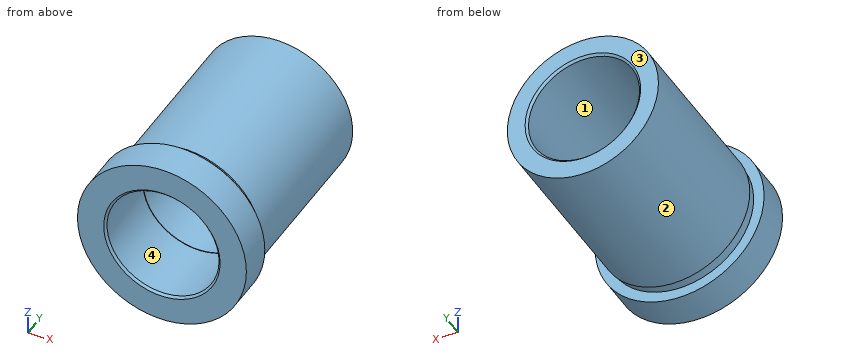
from build123d import *

# Parameters (mm, degrees)
CUT_EXTRUDE1_DEPTH      = 57.762663785
CUT_EXTRUDE1_DEPTH_BACK = 57.762663785
SKETCH2_R               = 12.5
SKETCH4_R               = 12.6
CUT_EXTRUDE2_DEPTH      = 16
CHAMFER4_SIZE           = 0.5
CHAMFER5_SIZE           = 0.5


with BuildPart() as part:
    # Sketch1 → Revolve1 (revolve)
    with BuildSketch(Plane.XY, mode=Mode.PRIVATE) as revolve1_sk:
        Polygon((0, 0), (19, 0), (19, 8), (16.65, 8), (16.65, 10.35), (17, 10.35), (17, 50), (0, 50), align=None)
    revolve(revolve1_sk.sketch.rotate(Axis((0, 50, 0), (0, -1, 0)), 180), axis=Axis((0, 50, 0), (0, -1, 0)))

    # Sketch2 → Cut-Extrude1 (cut, two sides: drawn at the far end of the back side and taken through both)
    with BuildSketch(Plane.XZ.offset(-CUT_EXTRUDE1_DEPTH_BACK)):
        Circle(SKETCH2_R)
    extrude(amount=CUT_EXTRUDE1_DEPTH + CUT_EXTRUDE1_DEPTH_BACK, mode=Mode.SUBTRACT)

    # Sketch4 → Cut-Extrude2 (cut)
    with BuildSketch(Plane.XZ):
        Circle(SKETCH4_R)
    extrude(amount=-CUT_EXTRUDE2_DEPTH, mode=Mode.SUBTRACT)

    # Chamfer4
    chamfer4_edges = [part.edges().sort_by_distance(p)[0] for p in [
        (-12.6, 0, 0),
    ]]
    chamfer(chamfer4_edges, length=CHAMFER4_SIZE)

    # Chamfer5
    chamfer5_edges = [part.edges().sort_by_distance(p)[0] for p in [
        (-12.5, 50, 0),
    ]]
    chamfer(chamfer5_edges, length=CHAMFER5_SIZE)


solid = part.part
Geometry: final body of the model. Coordinates: model frame, mm. Face numbers are marked on the shaded views. Round coordinates to 2 decimals unless told otherwise and drop trailing zeros. Order: outer loops, then holes, each group sorted by start corner. A loop starts at its lowest first (then second) coordinate and runs counter-clockwise, first axis right, second up.
Q1. Section D-D, the plane z = 16. Output: boundary loops of the cut face in (x, y).
Result sheet:
outline: (-10.25, 0) - (10.25, 0) - (10.25, 8) - (4.61, 8) - (4.61, 10.35) - (5.74, 10.35) - (5.74, 50) - (-5.74, 50) - (-5.74, 10.35) - (-4.61, 10.35) - (-4.61, 8) - (-10.25, 8) - close
Q2. Mould query, pull axis Z, two halves, no side actions, for the marked faces 1, 2, 3 and 4. Classes: released by +Z, released by -Z, zero draft, split by the parting line, or undercut.
Result sheet:
face 1: undercut
face 2: split by the parting line
face 3: zero draft
face 4: undercut
Q3. Section B-B, the plane z = 0. Output: boundary loops of the cut face in (x, y), and give its area (3 significant figures).
Result sheet:
outline: (-19, 0) - (-13.1, 0) - (-12.6, 0.5) - (-12.6, 16) - (-12.5, 16) - (-12.5, 49.5) - (-13, 50) - (-17, 50) - (-17, 10.35) - (-16.65, 10.35) - (-16.65, 8) - (-19, 8) - close; (12.5, 16) - (12.6, 16) - (12.6, 0.5) - (13.1, 0) - (19, 0) - (19, 8) - (16.65, 8) - (16.65, 10.35) - (17, 10.35) - (17, 50) - (13, 50) - (12.5, 49.5) - close
area: 477 mm2
Q4. Section A-A, the plane x = 0. Output: boundary loops of the cut face in (y, z), and give its area (3 significant figures).
Result sheet:
outline: (0, -19) - (8, -19) - (8, -16.65) - (10.35, -16.65) - (10.35, -17) - (50, -17) - (50, -13) - (49.5, -12.5) - (16, -12.5) - (16, -12.6) - (0.5, -12.6) - (0, -13.1) - close; (0, 13.1) - (0.5, 12.6) - (16, 12.6) - (16, 12.5) - (49.5, 12.5) - (50, 13) - (50, 17) - (10.35, 17) - (10.35, 16.65) - (8, 16.65) - (8, 19) - (0, 19) - close
area: 477 mm2
Q5. Material intervals for probe 1 along Z at (x, y) = (0, 7); probe 2 along Y at (x, z) = (16, -7.5); probe 3 along X at (y, z) = (37, -5.5), sorted ascending.
Result sheet:
probe 1: z = -19 to -12.6, 12.6 to 19
probe 2: y = 0 to 8
probe 3: x = -16.09 to -11.22, 11.22 to 16.09
Q6. Pin query (flat end, axial travel): pin 1 (1 mm diameter, centred on y = 17, z = -4, fed in from +X); pin 2 (8 mm diameter, centred on y = 42, z = 11, fed in from +X); pin 3 (1.5 mm diameter, centred on x = -10, y = 9.5, fed in from +Z). Return the tip coordinate at first contact, or that it passes through.
Result sheet:
pin 1: stops at x = 16.64
pin 2: stops at x = 15.49
pin 3: stops at z = 13.84
Q7. Section C-C, the plane y = 11. Output: boundary loops of the cut face in (x, z), and give its area (3 significant figures).
Result sheet:
outline: circle Ø34 at (0, 0); hole circle Ø25.2 at (0, 0)
area: 409 mm2
